Design review of the part built by this model. Coordinates are the model's own, in mm. Give positions to 0.01 mm unless a question says otherwise; leave off trailing zeros. Write each loop counter-clockwise with the first axis right and the second up, starting at its lowest first coordinate (ties: lowest second). Pieces come first, ordered by that corner, then holes. Notation, with made-up numbers: M 13.25,1.5 L 35.25,1.5 A25 cw 35.25,24.5 Z; hole C 41,38 d4. An arc over 180 degrees is marked long. Write each question's results on one line, items separated by ' | '. Start each with the question number.
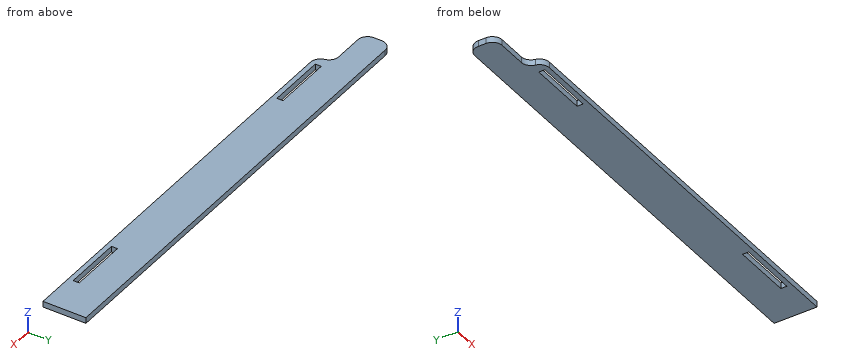
Autodesk Inventor part; units mm, degrees
ref_plane "YZ Plane" through (0, 0, 0) normal (1, 0, 0) x (0, 1, 0)
ref_plane "XZ Plane" through (0, 0, 0) normal (0, 1, 0) x (-1, 0, 0)
ref_plane "XY Plane" through (0, 0, 0) normal (0, 0, 1) x (1, 0, 0)
sketch "Sketch1" plane through (0, 0, 0) normal (0, 0, 1) x (1, 0, 0)
  line L0 (-120, -11) -> (120, -11)
  line L1 (120, -11) -> (120, 11)
  line L2 (120, 11) -> (-120, 11)
  line L3 (-120, 11) -> (-120, -11)
  line L4 (-120, -11) -> (120, 11) construction
  line L5 (120, -11) -> (-120, 11) construction
  line L6 (-90, -5.43) -> (-59.93, -5.43)
  line L7 (-59.93, -5.43) -> (-59.93, -8.5)
  line L8 (-59.93, -8.5) -> (-90, -8.5)
  line L9 (-90, -8.5) -> (-90, -5.43)
  line L10 (-90, -5.43) -> (-59.93, -8.5) construction
  line L11 (-59.93, -5.43) -> (-90, -8.5) construction
  line L12 (100.14, -5.42) -> (70.07, -5.42)
  line L13 (70.07, -5.42) -> (70.07, -8.5)
  line L14 (70.07, -8.5) -> (100.14, -8.5)
  line L15 (100.14, -8.5) -> (100.14, -5.42)
  line L16 (100.14, -5.42) -> (70.07, -8.5) construction
  line L17 (70.07, -5.42) -> (100.14, -8.5) construction
  line L18 (-120, -11) -> (-95, -11)
  line L19 (-95, -11) -> (-95, -3)
  line L20 (-95, -3) -> (-120, -3)
  line L21 (-120, -3) -> (-120, -11)
  point P0 (0, 0)
  point P1 (-74.965, -6.965)
  point P2 (85.105, -6.96)
  point P3 (-95, -11)
  dimension "d0" = 240
  dimension "d1" = 22
  dimension "d2" = 30.07
  dimension "d3" = 3.07
  dimension "d4" = 2.5
  dimension "d5" = 30
  dimension "d6" = 30.07
  dimension "d7" = 3.08
  dimension "d8" = 2.5
  dimension "d9" = 130
  dimension "d12" = 25
  dimension "d13" = 8
extrude "Plate1" add sketch "Sketch1" along normal blind 3 contours L19 L20 L3 L2 L1 L0
fillet "Corner Round1" radius 5 4 edges at (-120, 11, 1.5) (-120, -3, 1.5) (-95, -3, 1.5) (-95, -11, 1.5)
equation "\"d10\" = Thickness"
equation "\"BendRadius\" = Thickness"
equation "\"BendReliefWidth\" = Thickness"
equation "\"BendReliefDepth\" = 0.5 * Thickness"
equation "\"CornerReliefSize\" = 4 * Thickness"
equation "\"MinimumRemnant\" = 2 * Thickness"
equation "\"TransitionRadius\" = BendRadius"
equation "\"JacobiRadiusSize\" = BendRadius"
equation "\"GapSize\" = Thickness"
properties part number "Starting Path Wall"
Q1. For pin 1 Ø0.9 at (y, z) = (-6.5, 2) entering from -X, flat-tipped, find the tip position at first contact; note if it passes through.
Q2. We need section B-B on z = 0.8. Count the separate pieces of the cut face and the enclosed holes in it, and give its area (3 significant figures).
Q3. Wall thickness on line 1 along X through (y, z) = (-7.75, 1.2); line 2 along Y through (x, z) = (89, 0.8); line 3 along X through (y, z) = (-6.75, 1.1): over which ranges is each line inside the solid? List them lowest first. Write a range as from..to.
Q4. We need section A-A on x = 74.5. Write out the cut boundary in (y, z), and give its area (3 significant figures).
Answer sheet:
1) pin 1: x = -95.4
2) separate pieces: 1 | enclosed holes: 2 | area: 4,890 mm^2
3) line 1: -94.89..-90, -59.93..70.07, 100.14..120 | line 2: -11..-8.5, -5.42..11 | line 3: -95.16..-90, -59.93..70.07, 100.14..120
4) outline: M -11,0 L -8.5,0 L -8.5,3 L -11,3 Z; M -5.42,0 L 11,0 L 11,3 L -5.42,3 Z | area: 56.8 mm^2
